from build123d import *

# Parameters (mm, degrees)
SKETCH_1_W          = 40
SKETCH_1_H          = 35.45
EXTRUDE_1_DEPTH     = 20
FILLET_1_R          = 10
SKETCH_2_R          = 1.5
CUT_EXTRUDE_1_DEPTH = 77
SKETCH_3_W          = 2
SKETCH_3_H          = 10
EXTRUDE_2_DEPTH     = 3
SKETCH_4_W          = 13.504293884
SKETCH_4_H          = 10
CUT_EXTRUDE_2_DEPTH = 3
FILLET_2_R          = 1


with BuildPart() as part:
    # 草图1 → 凸台-拉伸1 (new body)
    with BuildSketch(Plane(origin=(0, 0, 0), x_dir=(1, 0, 0), z_dir=(0, 1, 0))):
        Rectangle(SKETCH_1_W, SKETCH_1_H)
    extrude(amount=EXTRUDE_1_DEPTH)

    # 圆角1
    fillet_1_edges = [part.edges().sort_by_distance(p)[0] for p in [
        (-20, 0, 0),
        (-20, 20, 0),
        (20, 0, 0),
        (20, 20, 0),
    ]]
    fillet(fillet_1_edges, radius=FILLET_1_R - 0.0001)  # a hair under: the kernel refuses the full size

    # 草图2 → 切除-拉伸1 (cut)
    with BuildSketch(Plane(origin=(0, 0, -17.725), x_dir=(-1, 0, 0), z_dir=(0, 0, -1))):
        with Locations((-10, 10)):
            Circle(SKETCH_2_R)
        with Locations((10, 10)):
            Circle(SKETCH_2_R)
    extrude(amount=-CUT_EXTRUDE_1_DEPTH, mode=Mode.SUBTRACT)

    # 草图3 → 凸台-拉伸2 (add)
    with BuildSketch(Plane(origin=(0, 0, -17.725), x_dir=(-1, 0, 0), z_dir=(0, 0, -1))):
        with Locations((-6, 5)):
            Rectangle(SKETCH_3_W, SKETCH_3_H)
        with Locations((-6, 15)):
            Rectangle(SKETCH_3_W, SKETCH_3_H)
        with Locations((-4, 5)):
            Rectangle(SKETCH_3_W, SKETCH_3_H)
        with Locations((-4, 15)):
            Rectangle(SKETCH_3_W, SKETCH_3_H)
    extrude(amount=EXTRUDE_2_DEPTH)

    # 草图4 → 切除-拉伸2 (cut)
    with BuildSketch(Plane(origin=(0, 0, -20.725), x_dir=(-1, 0, 0), z_dir=(0, 0, -1))):
        with Locations((-7, 10)):
            Rectangle(SKETCH_4_W, SKETCH_4_H)
    extrude(amount=-CUT_EXTRUDE_2_DEPTH, mode=Mode.SUBTRACT)

    # 圆角2
    fillet_2_edges = [part.edges().sort_by_distance(p)[0] for p in [
        (7, 17.5, -17.725),
        (3, 17.5, -17.725),
        (7, 2.5, -17.725),
        (3, 2.5, -17.725),
    ]]
    fillet(fillet_2_edges, radius=FILLET_2_R)


solid = part.part
Input: part model. Units: mm. Frame: model coordinates. A direction names the side the tool comes from. Coordinates: 2 decimals unless noted, no trailing zeros. Loops run counter-clockwise (first coordinate to the right, second up) from the corner with the lowest first, then second, coordinate; pieces in that order, holes last.
Q1. Set-up query: faces 5 (the face through (3, 17, -20)), 6 (the face through (-8.8, 9.1, -0.2)), 7 (the face through (7, 3, -20)). Return all of +Z, -Z, +X, -X, +Y, -Y with unobstructed straight access to the full face (end or side cutting, diameter ignored); none if empty.
Q2. Material intervals for line 1 (Y direction, x = 10, z = 3); line 2 (X direction, y = 9, z = 16); line 3 (Z direction, x = 8.5, y = 4.75) (3 decimals), sorted ascending.
Q3. Contact query for flat-ended pins moving along their axis: pin 1 (1.6 mm diameter, centred on y = 1.5, z = -20, fed in from +X); pin 2 (2 mm diameter, centred on y = 16.5, z = -19.5, fed in from -X); pin 3 (3.5 mm diameter, centred on x = 10, y = 10, fed in from -Z) (3 decimals). Output: stop coordinate, or through.
Q4. Cut plane C-C (y = 2). Output: boundary loops of the cut face in (x, z) (3 decimals).
Q5. Cut plane A-A (z = 10). Give the number of separate pieces and of enclosed holes in the cut face, then the cut area to 3 significant figures.
Q6. Cut plane D-D (x = 16.5). Output: boundary loops of the cut face in (y, z) (3 decimals), then the cut area to 3 significant figures.
Q7. Draft query along Y for faces 1 (the face through (7.3, 17.46, -18.01)), 2 (the face through (0, 20, -2)), 3 (the face through (11.2, 9.1, -0.2)), 4 (the face through (5, 15, -19)). Return one class per face: +Y half, -Y half, draft (parallel to the pull), parting line (faces both ways), or undercut.
Q8. Cut plane B-B (x = 4). Output: boundary loops of the cut face in (y, z) (3 decimals).
Working result:
1. face 5: -Z, -X, +Y, -Y
1. face 6: +Z, -Z
1. face 7: -Z, +X, +Y, -Y
2. line 1: y = 0 to 8.5, 11.5 to 20
2. line 2: x = -19.95 to -11.12, -8.88 to 8.88, 11.12 to 19.95
2. line 3: z = -17.725 to 17.725
3. pin 1: stops at x = 7
3. pin 2: stops at x = 2.97
3. pin 3: stops at z = -17.725
4. outline: (-16, -17.725) - (2, -17.725) arc R1 cw to (3, -18.725) - (3, -20.725) - (7, -20.725) - (7, -18.725) arc R1 cw to (8, -17.725) - (16, -17.725) - (16, 17.725) - (-16, 17.725) - close
5. separate pieces: 1
5. enclosed holes: 2
5. area: 700 mm2
6. outline: (2.401, -17.725) - (17.599, -17.725) - (17.599, 17.725) - (2.401, 17.725) - close
6. area: 539 mm2
7. face 1: draft
7. face 2: +Y half
7. face 3: undercut
7. face 4: undercut
8. outline: (0, -20.725) - (5, -20.725) - (5, -17.725) - (15, -17.725) - (15, -20.725) - (20, -20.725) - (20, 17.725) - (0, 17.725) - close
